Design review of the part built by this model. Coordinates are the model's own, in mm. A direction names the side the tool comes from. Coordinates: 2 decimals unless noted, no trailing zeros. Loops run counter-clockwise (first coordinate to the right, second up) from the corner with the lowest first, then second, coordinate; pieces in that order, holes last. Notation, with made-up numbers: (-39.75, -13) -> (19.25, -13) arc R34 ccw to (19.25, 17) -> close; hole circle Ø10 at (39.5, -17). An arc over 180 degrees is marked (long way). One line per item, written item: value. Start each with the question number.
1. Add section B-B on x = 3.5. Write out the cut boundary in (y, z).
2. Machinability: for faces 4 (the cylindrical face through (18.67, -4.21, 1.53)), 5 (the flat face through (6, -12.7, 6)), which of the approach directions +Z, -Z, +X, -X, +Y, -Y give a long, thin tool a straight path to every point of the face, cutting with its end or side? Answer none if there is none.
3. Insertion check: pin 1 (2 mm diameter, centred on y = -2, z = 20.5, fed in from +X); pin 2 (3 mm diameter, centred on x = 20.5, y = -3, fed in from +Z); pin 3 (1.5 mm diameter, centred on x = 7.5, y = -6.5, fed in from -Z). Each pin has a flat end and moves straight along its axis. Give the tip position at first contact, or say it passes through.
4. Add section A-A on y = -11.75. Write out the cut boundary in (x, z), plus the area to 3 significant figures.
5. Add section D-D on y = -6.35. Write out the cut boundary in (x, z), plus the area to 3 significant figures.
6. For probe 1 along X at (y, z) = (-6.35, 1.4); probe 2 along X at (y, z) = (-8.5, 2.5); probe 3 along X at (y, z) = (-2, 8), list the stretches that pass through material, from the lowest coordinate up.
7. Draft analysis for pull direction X (two halves, no side actions). For faces 1 (the flat face through (19.5, -12.7, 19.5)), 2 (the flat face through (25.4, -6, 13)), 3 (the flat face through (7, -6, 2.54)), state which applies: pulls with the +X half, pulls with the -X half, needs draft (parallel to the pull), parting line crosses it, or undercut.
8. Add section C-C on y = -3.25. Write out the cut boundary in (x, z).
```python
from build123d import *

# Parameters (mm, degrees)
F1_DEPTH    = 12.7
F2_R        = 2.54
F3_DEPTH    = 2.54
F4_T1_DEPTH = 51.5282991577
F4_T3_DEPTH = 51.5282991577


# Not quite as in the source:
# - a fillet or chamfer that OpenCascade refuses, or shapes differently, is made with other operations: its cross-section is extruded or revolved along the edge and cut away or added


with BuildPart() as f1:
    # F0 (on Front) → F1 (new body)
    with BuildSketch(Plane.XZ):
        with BuildLine():
            Line((0, 25.4), (0, 12.7))
            Line((0, 12.7), (8.89, 12.7))
            ThreePointArc((8.89, 12.7), (10.0059231637, 15.3940768363), (12.7, 16.51))
            Line((12.7, 16.51), (12.7, 25.4))
            Line((12.7, 25.4), (0, 25.4))
        make_face()
        with BuildLine():
            Line((16.51, 12.7), (25.4, 12.7))
            Line((25.4, 12.7), (25.4, 25.4))
            Line((25.4, 25.4), (12.7, 25.4))
            Line((12.7, 25.4), (12.7, 16.51))
            ThreePointArc((12.7, 16.51), (15.3940768363, 15.3940768363), (16.51, 12.7))
        make_face()
        with BuildLine():
            Line((12.7, 8.89), (12.7, 0))
            Line((12.7, 0), (25.4, 0))
            Line((25.4, 0), (25.4, 12.7))
            Line((25.4, 12.7), (16.51, 12.7))
            ThreePointArc((16.51, 12.7), (15.3940768363, 10.0059231637), (12.7, 8.89))
        make_face()
        with BuildLine():
            Line((0, 12.7), (0, 0))
            Line((0, 0), (12.7, 0))
            Line((12.7, 0), (12.7, 8.89))
            ThreePointArc((12.7, 8.89), (10.0059231637, 10.0059231637), (8.89, 12.7))
            Line((8.89, 12.7), (0, 12.7))
        make_face()
    extrude(amount=F1_DEPTH)

    # F2 (on Top) → F3 (cut)
    with BuildSketch(Plane.XY):
        with Locations((7.1409146445, -6.35)):
            Circle(F2_R)
        with Locations((17.3009146445, -6.35)):
            Circle(F2_R)
    extrude(amount=F3_DEPTH, mode=Mode.SUBTRACT)

    # F4: chamfer of 5.08 on 10 edges, made by hand

    # F4_s2 → F4_t1 (cut)
    with BuildSketch(Plane.XY.offset(-13.0641495789)):
        Polygon((0, -7.62), (5.08, -12.7), (0, -12.7), align=None)
        Polygon((20.32, -12.7), (25.4, -7.62), (25.4, -12.7), align=None)
        Polygon((0, -5.08), (5.08, 0), (0, 0), align=None)
        Polygon((20.32, 0), (25.4, -5.08), (25.4, 0), align=None)
    extrude(amount=F4_T1_DEPTH, mode=Mode.SUBTRACT)

    # F4_s4 → F4_t3 (cut)
    with BuildSketch(Plane.YZ.offset(-13.0641495789)):
        Polygon((-7.62, 0), (-12.7, 5.08), (-12.7, 0), align=None)
        Polygon((-7.62, 25.4), (-12.7, 20.32), (-12.7, 25.4), align=None)
        Polygon((-5.08, 0), (0, 5.08), (0, 0), align=None)
        Polygon((-5.08, 25.4), (0, 20.32), (0, 25.4), align=None)
    extrude(amount=F4_T3_DEPTH, mode=Mode.SUBTRACT)

    # F4_s5 → F4_t6 (revolve, cut)
    with BuildSketch(Plane.YZ.offset(12.7)):
        Polygon((-12.7, 3.81), (-7.62, 8.89), (-12.7, 8.89), align=None)
    revolve(axis=Axis((12.7, -12.7, 12.7), (0, 1, 0)), mode=Mode.SUBTRACT)

    # F4_s7 → F4_t8 (revolve, cut)
    with BuildSketch(Plane.YZ.offset(12.7)):
        Polygon((0, 3.81), (-5.08, 8.89), (0, 8.89), align=None)
    revolve(axis=Axis((12.7, 0, 12.7), (0, 1, 0)), mode=Mode.SUBTRACT)


solid = f1.part
```
Worked answers:
1. outline: (-11.12, 3.5) -> (-7.62, 0) -> (-5.08, 0) -> (-1.58, 3.5) -> (-1.58, 21.9) -> (-5.08, 25.4) -> (-7.62, 25.4) -> (-11.12, 21.9) -> close
2. face 4: -Z
2. face 5: +Z, -Z, +X, -X, -Y
3. pin 1: stops at x = 23.32
3. pin 2: stops at z = 24.82
3. pin 3: stops at z = 2.54
4. outline: (4.13, 4.13) -> (21.27, 4.13) -> (21.27, 21.27) -> (4.13, 21.27) -> close; hole circle Ø15.88 at (12.7, 12.7)
4. area: 95.7 mm²
5. outline: (0, 0) -> (4.6, 0) -> (4.6, 2.54) -> (9.68, 2.54) -> (9.68, 0) -> (14.76, 0) -> (14.76, 2.54) -> (19.84, 2.54) -> (19.84, 0) -> (25.4, 0) -> (25.4, 25.4) -> (0, 25.4) -> close; hole circle Ø7.62 at (12.7, 12.7)
5. area: 574 mm²
6. probe 1: x = 0 to 4.6, 9.68 to 14.76, 19.84 to 25.4
6. probe 2: x = 0.88 to 5.79, 8.49 to 15.95, 18.65 to 24.52
6. probe 3: x = 3.08 to 7.66, 17.74 to 22.32
7. face 1: needs draft
7. face 2: pulls with the +X half
7. face 3: undercut
8. outline: (1.83, 1.83) -> (23.57, 1.83) -> (23.57, 23.57) -> (1.83, 23.57) -> close; hole circle Ø11.28 at (12.7, 12.7)
